Read the model definition and answer for the solid it produces. Units are mm, in the model's axes. Face numbers are marked on the shaded views. A direction names the side the tool comes from. Round coordinates to 2 decimals unless told otherwise and drop trailing zeros. Loops run counter-clockwise (first coordinate to the right, second up) from the corner with the lowest first, then second, coordinate; pieces in that order, holes last. Notation, with made-up numbers: M -34,55.5 L -15,55.5 A26 cw -15,71.5 Z; hole C -1.5,47 d7. An arc over 180 degrees is marked long. Write each question's results on one line, items separated by ' | '.
```python
from build123d import *

# Parameters (mm, degrees)
F0_W          = 304.8
F0_H          = 533.4
F1_DEPTH      = 63.5
F1_DEPTH_BACK = 63.5
F3_DEPTH      = 127
F4_SIZE       = 12.7
F5_SIZE       = 5.08


# Not quite as in the source:
# - a feature names something its author has since deleted; it is built from what else it names


with BuildPart() as f1:
    # F0 (on Right) → F1 (new body, two sides)
    with BuildSketch(Plane.YZ) as f1_sk:
        Rectangle(F0_W, F0_H)
    extrude(amount=F1_DEPTH)
    extrude(f1_sk.sketch, amount=-F1_DEPTH_BACK)

    # F2 (on face) → F3 (cut, through all)
    with BuildSketch(Plane.YZ.offset(63.5)):
        Polygon((-114.3, 190.5), (-152.4, 190.5), (-152.4, 63.5), (-76.2, 63.5), align=None)
        Polygon((152.4, 190.5), (114.3, 190.5), (76.2, 63.5), (152.4, 63.5), align=None)
    extrude(amount=-F3_DEPTH, mode=Mode.SUBTRACT)

    # F4
    f4_edges = [f1.edges().sort_by_distance(p)[0] for p in [
        (63.5, 0, 266.7),
        (-63.5, 0, 266.7),
    ]]
    chamfer(f4_edges, length=F4_SIZE)

    # F5
    f5_edges = [f1.edges().sort_by_distance(p)[0] for p in [
        (63.5, -114.3, 63.5),
        (63.5, -95.25, 127),
        (63.5, -133.35, 190.5),
        (63.5, -152.4, 222.25),
        (57.15, -152.4, 260.35),
        (0, -152.4, 266.7),
        (-63.5, -152.4, 222.25),
        (0, -152.4, 190.5),
        (0, -152.4, 63.5),
        (-63.5, -114.3, 63.5),
        (-63.5, -95.25, 127),
        (-63.5, -133.35, 190.5),
        (-57.15, -152.4, 260.35),
        (-63.5, -152.4, -101.6),
        (0, -152.4, -266.7),
        (63.5, -152.4, -101.6),
        (-63.5, 0, -266.7),
        (63.5, 0, -266.7),
        (0, 152.4, -266.7),
        (63.5, 152.4, -101.6),
        (63.5, 114.3, 63.5),
        (63.5, 95.25, 127),
        (63.5, 133.35, 190.5),
        (63.5, 152.4, 222.25),
        (57.15, 152.4, 260.35),
        (0, 152.4, 266.7),
        (-57.15, 152.4, 260.35),
        (-63.5, 152.4, 222.25),
        (-63.5, 133.35, 190.5),
        (-63.5, 95.25, 127),
        (0, 152.4, 190.5),
        (-63.5, 114.3, 63.5),
        (0, 152.4, 63.5),
        (-63.5, 152.4, -101.6),
    ]]
    chamfer(f5_edges, length=F5_SIZE)


solid = f1.part
```
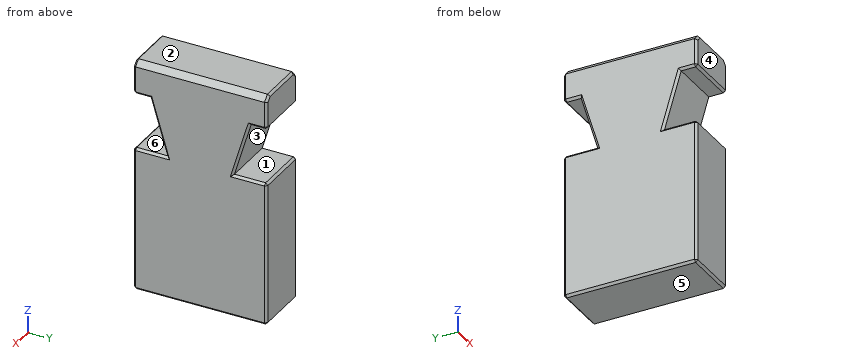
1. Given P1, Ø2, axis at x = 36, z = 128, coming from the -Y side, flat-ended and moving along its own axis, determine where the tip first touches the part or whether it passes through.
Completed:
P1: stops at y = -95.85
2. Find section A-A, the plane x = 19. Give the vertices of the cut face in (y, z).
Completed:
outline: M -152.4,-261.62 L -147.32,-266.7 L 147.32,-266.7 L 152.4,-261.62 L 152.4,58.42 L 147.32,63.5 L 76.2,63.5 L 114.3,190.5 L 147.32,190.5 L 152.4,195.58 L 152.4,261.62 L 147.32,266.7 L -147.32,266.7 L -152.4,261.62 L -152.4,195.58 L -147.32,190.5 L -114.3,190.5 L -76.2,63.5 L -147.32,63.5 L -152.4,58.42 Z
3. Find section B-B, the plane y = -89. Give the vertices of the cut face in (x, z), then the cut area to 3 significant figures.
Completed:
outline: M -63.5,-261.62 L -58.42,-266.7 L 58.42,-266.7 L 63.5,-261.62 L 63.5,58.42 L 58.42,63.5 L -58.42,63.5 L -63.5,58.42 Z; M -63.5,123.85 L -58.42,106.17 L 58.42,106.17 L 63.5,123.85 L 63.5,254 L 50.8,266.7 L -50.8,266.7 L -63.5,254 Z | area: 62,000 mm2
4. Find section C-C, the plane y = 99. Give the vertices of the cut face in (x, z).
Completed:
outline: M -63.5,-261.62 L -58.42,-266.7 L 58.42,-266.7 L 63.5,-261.62 L 63.5,58.42 L 58.42,63.5 L -58.42,63.5 L -63.5,58.42 Z; M -63.5,157.18 L -58.42,139.5 L 58.42,139.5 L 63.5,157.18 L 63.5,254 L 50.8,266.7 L -50.8,266.7 L -63.5,254 Z
5. Find the intervals of material crossed by L1, parallel to Z at x = 1, y = -119; L2, parallel to X at y = 81.5, z = 94; L3, parallel to Z at x = 57, y = 1, in increasing order.
Completed:
L1: z = -266.7 to 63.5, 190.5 to 266.7 | L2: x = -62.11 to 62.11 | L3: z = -266.7 to 260.5
6. Which of the six approach directions +Z, -Z, +X, -X, +Y, -Y give full straight-line access (tool end or side, diameter ignored) to the marked faces 5 and 6?
Completed:
face 5: -Z, +X, -X, +Y, -Y | face 6: +X, -X, -Y
7. Determine the mould class of the marked faces 1, 2, 3 and 4 for opening direction Z: released by +Z, released by -Z, zero draft, split by the parting line, or undercut.
Completed:
face 1: undercut | face 2: released by +Z | face 3: undercut | face 4: zero draft
